from build123d import *

# Parameters (mm, degrees)
SKETCH1_R           = 1.25
BOSS_EXTRUDE1_DEPTH = 10
CUT_EXTRUDE1_REACH  = 94.193
SKETCH2_R           = 3
SKETCH3_R           = 7.5
SKETCH3_R_2         = 3
BOSS_EXTRUDE2_DEPTH = 3


with BuildPart() as part:
    # Sketch1 → Boss-Extrude1 (new body)
    with BuildSketch(Plane.XY):
        with BuildLine():
            Line((0.25, -3.240370349), (0.25, -41.740370349))
            Line((0.25, -41.740370349), (8.25, -85.075157412))
            ThreePointArc((8.25, -85.075157412), (10.208936196, -88.421482437), (13.855284626, -89.740370349))
            Line((13.855284626, -89.740370349), (18.855284626, -89.740370349))
            Line((18.855284626, -89.740370349), (18.855284626, -86.740370349))
            Line((18.855284626, -86.740370349), (13.855284626, -86.740370349))
            ThreePointArc((13.855284626, -86.740370349), (12.129255683, -86.116622764), (11.200712952, -84.533573379))
            Line((11.200712952, -84.533573379), (3.25, -41.740370349))
            Line((3.25, -41.740370349), (3.25, 0))
            ThreePointArc((3.25, 0), (-2.384848004, 2.207940217), (0.25, -3.240370349))
        make_face()
        Circle(SKETCH1_R, mode=Mode.SUBTRACT)
    extrude(amount=BOSS_EXTRUDE1_DEPTH)

    # Sketch2 → Cut-Extrude1 (cut, up to next)
    with BuildSketch(Plane.ZY.offset(-0.25), mode=Mode.PRIVATE) as cut_extrude1_sk1:
        with Locations(Location((5, -30.5, 0), (0, 0, 270))):
            Circle(SKETCH2_R)
    cut_extrude1_tool1 = extrude(cut_extrude1_sk1.sketch, amount=-CUT_EXTRUDE1_REACH, mode=Mode.PRIVATE) & part.part
    add(cut_extrude1_tool1.solids().sort_by_distance((0.25, -30.5, 5))[0], mode=Mode.SUBTRACT)

    # Sketch3 → Boss-Extrude2 (add)
    with BuildSketch(Plane.ZY.offset(-0.25)):
        with Locations((5, -30.5)):
            Circle(SKETCH3_R)
        with Locations(Location((5, -30.5, 0), (0, 0, 270))):
            Circle(SKETCH3_R_2, mode=Mode.SUBTRACT)
    extrude(amount=-BOSS_EXTRUDE2_DEPTH)


solid = part.part
Build history of the part. All positions in model axes, mm. A direction names the side the tool comes from. Give positions to 0.01 mm unless a question says otherwise; leave off trailing zeros. Order: outer loops, then holes, each group sorted by start corner. A loop starts at its lowest first (then second) coordinate and runs counter-clockwise, first axis right, second up. Notation, with made-up numbers: M 35,61.5 L 90,61.5 A32 cw 90,97.5 Z; hole C -38.75,-3.75 d8. An arc over 180 degrees is marked long. Put each result on its own line as item: value.
Item 1: 3-axis set-ups, long thin cutter, end or side, ignore diameter. For faces 1 (the flat face through (3.25, -21, 5)), 2 (the flat face through (0.25, -22, 5)), 3 (the flat face through (1, -8, 0)): which of +Z, -Z, +X, -X, +Y, -Y reach the whole face in a straight line?
From the geometry:
face 1: +Z, -Z, +X, +Y
face 2: +Z, -Z, -X, -Y
face 3: -Z, +X, -X, +Y
Item 2: Flat gauge pins, fed straight in: pin 1 Ø8 at (y, z) = (-63.5, 1) entering from +X; pin 2 Ø7 at (x, y) = (0.5, -4) entering from -Z; pin 3 Ø4 at (y, z) = (-34.5, 10) entering from +X. Where does each tip first touch, or does it go through?
From the geometry:
pin 1: stops at x = 8.04
pin 2: stops at z = 0
pin 3: stops at x = 3.25
Item 3: Slice it at A-A, the plane z = 5. Write the cut outline in (x, y), plus the area to 3 significant figures.
From the geometry:
outline: M 0.25,-41.74 L 8.25,-85.08 A5.7 ccw 13.86,-89.74 L 18.86,-89.74 L 18.86,-86.74 L 13.86,-86.74 A2.7 cw 11.2,-84.53 L 3.25,-41.74 L 3.25,-33.5 L 0.25,-33.5 Z; M 0.25,-27.5 L 3.25,-27.5 L 3.25,0 A3.25 ccw long 0.25,-3.24 Z; hole C 0,0 d2.5
area: 291 mm2
Item 4: Probe line 1 (Z direction, x = 2.3, y = -30.5); line 2 (X direction, y = -40, z = 1); line 3 (Y direction, x = 15.25, z = 4.5). List the from-to ranges inside material, lowest first. Write a range as [from, to].
From the geometry:
line 1: z = [-2.5, 2], [8, 12.5]
line 2: x = [0.25, 3.25]
line 3: y = [-89.74, -86.74]
Item 5: Two-plate mould, pull along X, no slides. Class faces 4 (the cylindrical face through (-0.27, -1.22, 4.93)), 5 (the cylindrical face through (12, -86, 5)), 6 (the flat face through (1, -8, 10)): +X half, -X half, draft (parallel to the pull), parting line (faces both ways), or undercut.
From the geometry:
face 4: undercut
face 5: +X half
face 6: draft
Item 6: Slice it at B-B, the plane y = -30.5. Write the cut outline in (x, z).
From the geometry:
outline: M 0.25,-2.5 L 3.25,-2.5 L 3.25,2 L 0.25,2 Z; M 0.25,8 L 3.25,8 L 3.25,12.5 L 0.25,12.5 Z
Item 7: Slice it at D-D, the plane y = -70. Write the cut outline in (x, z).
From the geometry:
outline: M 5.47,0 L 8.5,0 L 8.5,10 L 5.47,10 Z
Item 8: Slice it at C-C, the plane x = 16.5. Write the cut outline in (y, z), plus the area to 3 significant figures.
From the geometry:
outline: M -89.74,0 L -86.74,0 L -86.74,10 L -89.74,10 Z
area: 30.0 mm2
